Could you check a few things on this model? Use its own coordinates, in mm. Face numbers are marked on the shaded views. A direction names the side the tool comes from. Give positions to 0.01 mm unless a question says otherwise; leave off trailing zeros. Order: outer loops, then holes, each group sorted by start corner. A loop starts at its lowest first (then second) coordinate and runs counter-clockwise, first axis right, second up. Notation, with made-up numbers: M -21,-1.5 L 36,-1.5 A22 cw 36,36.5 Z; hole C 47,88.25 d3. An arc over 180 degrees is marked long. Return JSON: item names as keys, results as strings. Group by question number.
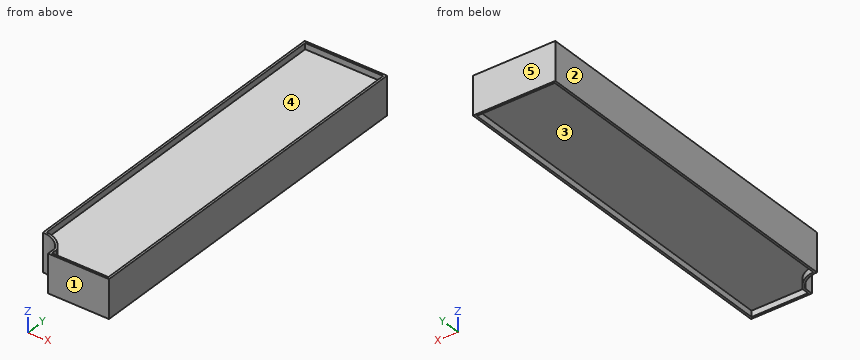
```python
from build123d import *

# Parameters (mm, degrees)
SKETCH1_W           = 191.44
SKETCH1_H           = 851.41
BOSS_EXTRUDE1_DEPTH = 89
CUT_EXTRUDE1_DEPTH  = 89
CUT_EXTRUDE2_DEPTH  = 14


with BuildPart() as part:
    # Sketch1 → Boss-Extrude1 (new body)
    with BuildSketch(Plane.XY):
        with Locations((95.72, 425.705)):
            Rectangle(SKETCH1_W, SKETCH1_H)
    extrude(amount=BOSS_EXTRUDE1_DEPTH)

    # Sketch2 → Cut-Extrude1 (cut)
    with BuildSketch(Plane.XY.offset(89)):
        with BuildLine():
            Line((50, 0), (50, 20))
            ThreePointArc((50, 20), (29.154759474, 41.924599124), (0, 50))
            Line((0, 50), (-42.502715258, 50))
            Line((-42.502715258, 50), (0, -54.761569713))
            Line((0, -54.761569713), (50, 0))
        make_face()
    extrude(amount=-CUT_EXTRUDE1_DEPTH, mode=Mode.SUBTRACT)

    # Sketch3 → Cut-Extrude2 (cut)
    with BuildSketch(Plane.XY.offset(89)):
        with BuildLine():
            Line((55, 21.222000884), (55, 5))
            Line((55, 5), (186.44, 5))
            Line((186.44, 5), (186.44, 846.41))
            Line((186.44, 846.41), (5, 846.41))
            Line((5, 846.41), (5, 54.796963049))
            ThreePointArc((5, 54.796963049), (34.377602026, 44.528628593), (55, 21.222000884))
        make_face()
    cut_extrude2 = extrude(amount=-CUT_EXTRUDE2_DEPTH, mode=Mode.SUBTRACT)

    # Mirror1: Cut-Extrude2 across plane
    add(cut_extrude2.mirror(Plane.XY.offset(44.5)), mode=Mode.SUBTRACT)


solid = part.part
```
1. Imagine slicing it at B-B, the plane x = 127. Please give me the cut outline in (y, z), plus the area to 3 significant figures.
2. If we mould it in two halves opening along Y, with no side actions, what happens to the marked faces 1, 2 and 3? For each: pulls with the +Y half, pulls with the -Y half, needs draft (parallel to the pull), parting line crosses it, or undercut.
3. Imagine slicing it at A-A, the plane y = 661. Please give me the cut outline in (x, z).
4. I need wall thicknesses on L1, parallel to X at y = 161, z = 83.5; L2, parallel to Y at x = 150.5, z = 13.5; L3, parallel to Z at x = 83, y = 240. Which ranges of each line are inside material? Lowest first, please. Write a range as from..to.
5. For pin 1 (6 mm diameter, centred on x = 30, z = 42.5, fed in from -Y); pin 2 (10 mm diameter, centred on y = 13.5, z = 58, fed in from -X); pin 3 (10 mm diameter, centred on x = 111, y = 333, fed in from -Z); pin 4 (4 mm diameter, centred on x = 122.5, z = 79, fed in from -Y), each with a flat end and sliding along its axis, tell me the tip position at first contact or that it passes through.
6. Which directions (+Z, -Z, +X, -X, +Y, -Y) give clear straight access to the entire face, cutting with the end or side of a thin tool? Please do the marked faces 4 and 5.
Values:
{
 "1": {"outline": "M 0,0 L 5,0 L 5,14 L 846.41,14 L 846.41,0 L 851.41,0 L 851.41,89 L 846.41,89 L 846.41,75 L 5,75 L 5,89 L 0,89 Z", "area": "52,200 mm²"},
 "2": {"face 1": "pulls with the -Y half", "face 2": "needs draft", "face 3": "undercut"},
 "3": {"outline": "M 0,0 L 5,0 L 5,14 L 186.44,14 L 186.44,0 L 191.44,0 L 191.44,89 L 186.44,89 L 186.44,75 L 5,75 L 5,89 L 0,89 Z"},
 "4": {"L1": "x = 0..5, 186.44..191.44", "L2": "y = 0..5, 846.41..851.41", "L3": "z = 14..75"},
 "5": {"pin 1": "stops at y = 39.4", "pin 2": "stops at x = 50", "pin 3": "stops at z = 14", "pin 4": "stops at y = 0"},
 "6": {"face 4": "+Z", "face 5": "+Z, -Z, +X, -X, +Y"}
}
